```python
from build123d import *

# Parameters (mm, degrees)
BOSS_EXTRUDE1_DEPTH            = 20
F_2_0MM_DOWEL_HOLE1_AT_2_COUNT = 2
F_2_0MM_DOWEL_HOLE1_AT_2_PITCH = 10
SKETCH8_R                      = 3.75
BOSS_EXTRUDE2_DEPTH            = 10
SKETCH9_W                      = 35
SKETCH9_H                      = 50
BOSS_EXTRUDE3_DEPTH            = 2.5
SKETCH10_W                     = 35
SKETCH10_H                     = 50
BOSS_EXTRUDE4_DEPTH            = 2.5
SKETCH11_W                     = 35
SKETCH11_H                     = 25
BOSS_EXTRUDE5_DEPTH            = 100
BOSS_EXTRUDE6_DEPTH            = 5
BOSS_EXTRUDE9_DEPTH            = 40
BOSS_EXTRUDE10_DEPTH           = 40
SKETCH24_W                     = 50
SKETCH24_H                     = 20
CUT_EXTRUDE4_DEPTH             = 5
SKETCH26_W                     = 40
SKETCH26_H                     = 20
CUT_EXTRUDE5_DEPTH             = 35
F_2_0MM_DOWEL_HOLE2_D          = 2
F_2_0MM_DOWEL_HOLE2_DEPTH      = 10
F_2_0MM_DOWEL_HOLE2_TIP        = 0.600860619
SKETCH30_R                     = 3.75
BOSS_EXTRUDE11_DEPTH           = 10


with BuildPart() as part:
    # Sketch1 → Boss-Extrude1 (new body)
    with BuildSketch(Plane(origin=(0, 0, 0), x_dir=(1, 0, 0), z_dir=(0, 1, 0))):
        Polygon((-12.5, 25), (-12.5, 20), (17.5, 20), (17.5, -20), (-12.5, -20), (-12.5, -25), (22.5, -25), (22.5, 25), align=None)
    extrude(amount=BOSS_EXTRUDE1_DEPTH)

    # Sketch7 → Ø2.0mm Dowel Hole1 (revolve, cut)
    with BuildSketch(Plane(origin=(-12.5, 15, -22.5), x_dir=(0, 0, 1), z_dir=(0, 1, 0))):
        Polygon((0, 0), (0, 10.600860619), (1, 10), (1, 0), align=None)
    f_2_0mm_dowel_hole1 = revolve(axis=Axis((-18.85, 15, -22.5), (1, 0, 0)), mode=Mode.SUBTRACT)

    # Ø2.0mm Dowel Hole1 at 2: Ø2.0mm Dowel Hole1 ×2
    with Locations(*[(0, -i * F_2_0MM_DOWEL_HOLE1_AT_2_PITCH, 0) for i in range(1, F_2_0MM_DOWEL_HOLE1_AT_2_COUNT)]):
        add(f_2_0mm_dowel_hole1, mode=Mode.SUBTRACT)

    # Mirror1: Ø2.0mm Dowel Hole1 across plane
    add(f_2_0mm_dowel_hole1.mirror(Plane.XY), mode=Mode.SUBTRACT)

    # Mirror1 copy 1 sketch → Mirror1 copy 1 (revolve, cut)
    with BuildSketch(Plane(origin=(-12.5, 5, 22.5), x_dir=(0, 0, -1), z_dir=(0, 1, 0))):
        Polygon((0, 0), (0, -10.600860619), (1, -10), (1, 0), align=None)
    revolve(axis=Axis((-18.85, 5, 22.5), (-1, 0, 0)), mode=Mode.SUBTRACT)

    # Sketch8 → Boss-Extrude2 (add)
    with BuildSketch(Plane(origin=(22.5, 0, 0), x_dir=(0, 0, -1), z_dir=(1, 0, 0))):
        with Locations((-10, 10)):
            Circle(SKETCH8_R)
    extrude(amount=BOSS_EXTRUDE2_DEPTH)

    # Sketch9 → Boss-Extrude3 (add)
    with BuildSketch(Plane(origin=(0, 20, 0), x_dir=(1, 0, 0), z_dir=(0, 1, 0))):
        with Locations((5, 0)):
            Rectangle(SKETCH9_W, SKETCH9_H)
    extrude(amount=BOSS_EXTRUDE3_DEPTH)

    # Sketch10 → Boss-Extrude4 (add)
    with BuildSketch(Plane.XZ):
        with Locations((5, 0)):
            Rectangle(SKETCH10_W, SKETCH10_H)
    extrude(amount=BOSS_EXTRUDE4_DEPTH)

    # Sketch11 → Boss-Extrude5 (add)
    with BuildSketch(Plane(origin=(0, 0, -25), x_dir=(-1, 0, 0), z_dir=(0, 0, -1))):
        with Locations((-5, 10)):
            Rectangle(SKETCH11_W, SKETCH11_H)
    extrude(amount=BOSS_EXTRUDE5_DEPTH)

    # Sketch12 → Boss-Extrude6 (add)
    with BuildSketch(Plane.ZY.offset(12.5)):
        Polygon((25, 22.5), (-125, 22.5), (-125, -2.5), (25, -2.5), (25, 0), (20, 0), (-20, 0), (-25, 0), (-25, 20), (-20, 20), (20, 20), (25, 20), align=None)
    extrude(amount=BOSS_EXTRUDE6_DEPTH)

    # Sketch20 → Boss-Extrude9 (add)
    with BuildSketch(Plane(origin=(22.5, 0, 0), x_dir=(0, 0, -1), z_dir=(1, 0, 0))):
        with BuildLine():
            ThreePointArc((125, -2.5), (137.5, 10), (125, 22.5))
            Line((125, 22.5), (125, -2.5))
        make_face()
    extrude(amount=-BOSS_EXTRUDE9_DEPTH)

    # Sketch23 → Boss-Extrude10 (add)
    with BuildSketch(Plane(origin=(22.5, 0, 0), x_dir=(0, 0, -1), z_dir=(1, 0, 0))):
        with BuildLine():
            Line((-25, -2.5), (-25, 22.5))
            ThreePointArc((-25, 22.5), (-37.5, 10), (-25, -2.5))
        make_face()
    extrude(amount=-BOSS_EXTRUDE10_DEPTH)

    # Sketch24 → Cut-Extrude4 (cut)
    with BuildSketch(Plane(origin=(22.5, 0, 0), x_dir=(0, 0, -1), z_dir=(1, 0, 0))):
        with Locations((100, 10)):
            Rectangle(SKETCH24_W, SKETCH24_H)
    extrude(amount=-CUT_EXTRUDE4_DEPTH, mode=Mode.SUBTRACT)

    # Sketch26 → Cut-Extrude5 (cut)
    with BuildSketch(Plane(origin=(22.5, 0, 0), x_dir=(0, 0, -1), z_dir=(1, 0, 0))):
        with Locations((100, 10)):
            Rectangle(SKETCH26_W, SKETCH26_H)
    extrude(amount=-CUT_EXTRUDE5_DEPTH, mode=Mode.SUBTRACT)

    # Ø2.0mm Dowel Hole2
    with Locations(Plane(origin=(17.5, 0, 0), x_dir=(0, 0, -1), z_dir=(1, 0, 0))):
        with Locations((77.5, 15), (77.5, 5), (122.5, 15), (122.5, 5)):
            Hole(F_2_0MM_DOWEL_HOLE2_D / 2, depth=F_2_0MM_DOWEL_HOLE2_DEPTH)
            with Locations((0, 0, -(F_2_0MM_DOWEL_HOLE2_DEPTH + F_2_0MM_DOWEL_HOLE2_TIP / 2))):  # 118° drill point
                Cone(0, F_2_0MM_DOWEL_HOLE2_D / 2, F_2_0MM_DOWEL_HOLE2_TIP, mode=Mode.SUBTRACT)

    # Sketch30 → Boss-Extrude11 (add)
    with BuildSketch(Plane.ZY.offset(17.5)):
        with Locations((-110, 10)):
            Circle(SKETCH30_R)
    extrude(amount=BOSS_EXTRUDE11_DEPTH)


solid = part.part
```
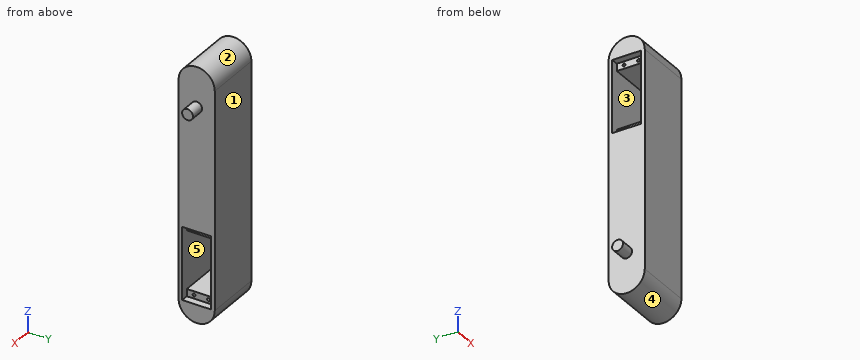
Build history of the part. All positions in model axes, mm. Face numbers are marked on the shaded views. A direction names the side the tool comes from. Give positions to 0.01 mm unless a question says otherwise; leave off trailing zeros. Loops run counter-clockwise (first coordinate to the right, second up) from the corner with the lowest first, then second, coordinate; pieces in that order, holes last. Notation, with made-up numbers: (8, -10) -> (56, -10) arc R26 ccw to (56, 20) -> close; hole circle Ø1 at (66, 37). An arc over 180 degrees is marked (long way). One line per question, with ' | ' between items.
Q1. Drill centre lines: line 1 along Z through (x, y) = (-5, 9.25); line 2 along Y through (x, z) = (11.75, -77.5); line 3 along Y through (x, z) = (-8, 22). Where is each one in solid material? Low to high. Write a range as [from, to].
Filled sheet:
line 1: z = [-137.48, -120], [-80, -20], [20, 37.48] | line 2: y = [-2.5, 4], [6, 14], [16, 22.5] | line 3: y = [-2.5, 4.13], [5.87, 14.13], [15.87, 22.5]
Q2. Drop flat-ended pins along their axis: pin 1 (2.5 mm diameter, centred on y = 15, z = 22.5, fed in from -X); pin 2 (4 mm diameter, centred on y = 11, z = 2, fed in from +X); pin 3 (1.6 mm diameter, centred on y = 15, z = -122.5, fed in from +X). Give the stop position or say it passes through.
Filled sheet:
pin 1: stops at x = -12.5 | pin 2: stops at x = 22.5 | pin 3: stops at x = 7.38
Q3. Pull direction Z, two halves, no side cores. Call the marked faces 1, 2 and 3: pulls with the +Z half, pulls with the -Z half, needs draft (parallel to the pull), parting line crosses it, or undercut.
Filled sheet:
face 1: needs draft | face 2: pulls with the +Z half | face 3: undercut
Q4. Cut at B-B, the plane z = 10. Write the cut outline in (x, y).
Filled sheet:
outline: (-17.5, -2.5) -> (22.5, -2.5) -> (22.5, 6.25) -> (32.5, 6.25) -> (32.5, 13.75) -> (22.5, 13.75) -> (22.5, 22.5) -> (-17.5, 22.5) -> (-17.5, 20) -> (17.5, 20) -> (17.5, 0) -> (-17.5, 0) -> close
Q5. Tool access for the marked faces 4 and 5: list every direction of +Z, -Z, +X, -X, +Y, -Y with a clear straight run to the whole face (end or side of a thin tool).
Filled sheet:
face 4: -Z, +X, -X | face 5: +X
Q6. Cut at A-A, the plane x = -9. Write the cut outline in (y, z).
Filled sheet:
outline: (-2.5, -125) arc R12.5 ccw to (22.5, -125) -> (22.5, 25) arc R12.5 ccw to (-2.5, 25) -> close; hole (0, -120) -> (20, -120) -> (20, -80) -> (0, -80) -> close; hole (0, -20) -> (20, -20) -> (20, 20) -> (0, 20) -> close; hole circle Ø2 at (5, -22.5); hole circle Ø2 at (5, 22.5); hole circle Ø2 at (15, -22.5); hole circle Ø2 at (15, 22.5)
Q7. Cut at C-C, the plane y = 10. Write the cut outline in (x, z).
Filled sheet:
outline: (-27.5, -113.75) -> (-17.5, -113.75) -> (-17.5, -137.5) -> (22.5, -137.5) -> (22.5, -125) -> (17.5, -125) -> (17.5, -120) -> (-12.5, -120) -> (-12.5, -80) -> (17.5, -80) -> (17.5, -75) -> (22.5, -75) -> (22.5, 6.25) -> (32.5, 6.25) -> (32.5, 13.75) -> (22.5, 13.75) -> (22.5, 37.5) -> (-17.5, 37.5) -> (-17.5, 25) -> (-12.5, 25) -> (-12.5, 20) -> (17.5, 20) -> (17.5, -20) -> (-12.5, -20) -> (-12.5, -25) -> (-17.5, -25) -> (-17.5, -106.25) -> (-27.5, -106.25) -> close
Q8. Cut at D-D, the plane z = -92.5. Write the cut outline in (x, y), plus the area to 3 significant figures.
Filled sheet:
outline: (-17.5, -2.5) -> (22.5, -2.5) -> (22.5, 0) -> (-12.5, 0) -> (-12.5, 20) -> (22.5, 20) -> (22.5, 22.5) -> (-17.5, 22.5) -> close | area: 300 mm²
